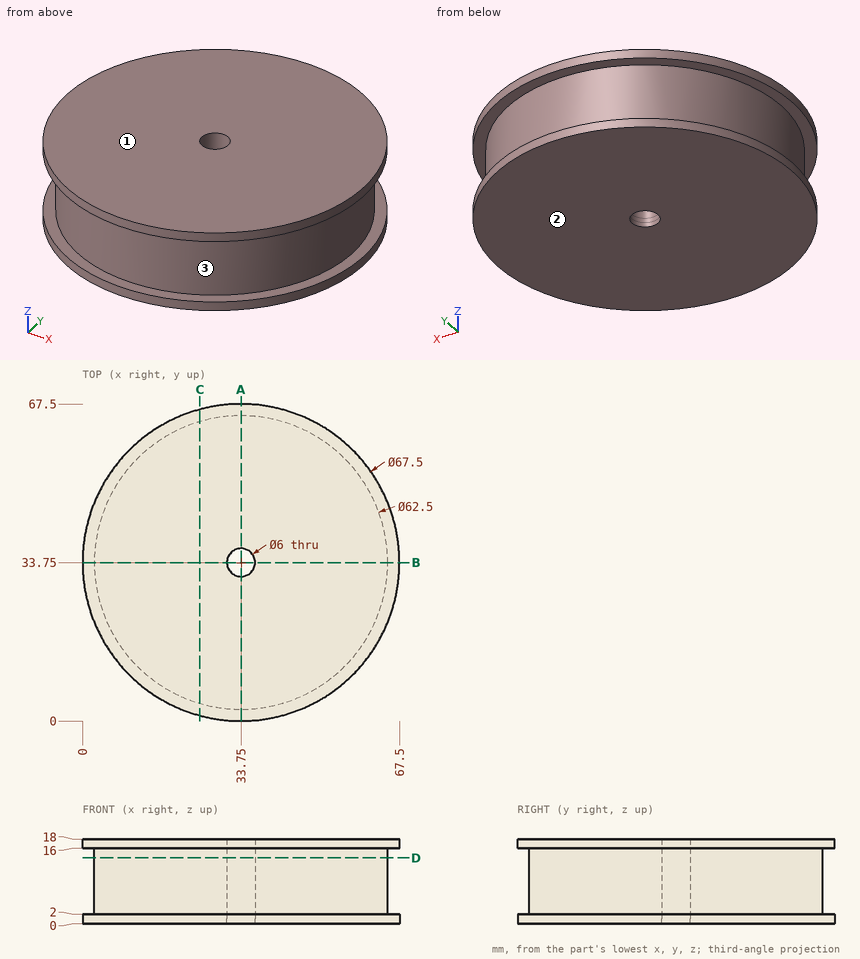
The drawing under review shows one solid part. Ordinate dimensions are in mm from its lowest x, y, z. Coordinates: 2 decimals unless noted, no trailing zeros. Loops run counter-clockwise (first coordinate to the right, second up) from the corner with the lowest first, then second, coordinate; pieces in that order, holes last. Notation, with made-up numbers: (48.25, 8) - (93.25, 8) arc R27 ccw to (93.25, 43) - close; hole circle Ø6 at (-23.5, 25). An arc over 180 degrees is marked (long way). Use CSV: the item, a comma, the result in double quotes. Start each with the question number.
1. Mouldability with a two-part tool opening along Z and no side actions: class the marked faces 1, 2 and 3 as released by +Z, released by -Z, zero draft, split by the parting line, or undercut.
2. To check wall thickness, follow probe 1 along Y at (x, z) = (33.5, 10.25); probe 2 along Y at (x, z) = (33.75, 0.4). State the ranges of each line that lie inside material, in increasing order.
3. Clearance check with flat-ended pins moving along their axes: pin 1 (3 mm diameter, centred on x = 43, z = 9, fed in from +Y); pin 2 (10 mm diameter, centred on y = 34, z = 8, fed in from -X); pin 3 (1.5 mm diameter, centred on y = 13.5, z = 13, fed in from +X); pin 4 (5 mm diameter, centred on x = 33.75, y = 33.75, fed in from -Z). State where each tip first meets the part, or that it passes through.
4. Add section C-C on x = 25. Give the boundary of the cut face in (y, z).
5. Add section A-A on x = 33.75. Give the boundary of the cut face in (y, z).
6. Add section D-D on z = 14. Give the boundary of the cut face in (x, y).
Resolved:
1,face 1,"released by +Z"
1,face 2,"released by -Z"
1,face 3,"undercut"
2,probe 1,"2.5 to 30.76, 36.74 to 65"
2,probe 2,"0 to 30.75, 36.75 to 67.5"
3,pin 1,"y = 64.02"
3,pin 2,"x = 2.5"
3,pin 3,"x = 58.17"
3,pin 4,"through"
4,outline,"(1.15, 0) - (66.35, 0) - (66.35, 2) - (63.75, 2) - (63.75, 16) - (66.35, 16) - (66.35, 18) - (1.15, 18) - (1.15, 16) - (3.75, 16) - (3.75, 2) - (1.15, 2) - close"
5,outline,"(0, 0) - (30.75, 0) - (30.75, 18) - (0, 18) - (0, 16) - (2.5, 16) - (2.5, 2) - (0, 2) - close; (36.75, 0) - (67.5, 0) - (67.5, 2) - (65, 2) - (65, 16) - (67.5, 16) - (67.5, 18) - (36.75, 18) - close"
6,outline,"circle Ø62.5 at (33.75, 33.75); hole circle Ø6 at (33.75, 33.75)"
